Design review of the part built by this model. Coordinates are the model's own, in mm. A direction names the side the tool comes from. Round coordinates to 2 decimals unless told otherwise and drop trailing zeros. Loops run counter-clockwise (first coordinate to the right, second up) from the corner with the lowest first, then second, coordinate; pieces in that order, holes last. Notation, with made-up numbers: (59.5, 8.5) - (88.5, 8.5) arc R32 cw to (88.5, 43.5) - close; hole circle Ø9 at (-12, 44). An arc over 180 degrees is marked (long way). Answer as CSV lines item,"result". Start each with the question number.
(1) Consider section A-A (x = 11.5). Give the boundary of the cut face in (y, z).
(2) Consider section B-B (z = -3.5). Give the boundary of the cut face in (x, y).
(3) Wall thickness on L1, parallel to Z at x = -39, y = 2.75; L2, parallel to Z at x = 18, y = 3.25; L3, parallel to Z at x = 41, y = 6.75: over which ranges is each line inside the solid? List them lowest first.
(4) Consider section D-D (y = 10). Count the separate pieces of the cut face and the enclosed holes in it, and give its area (3 significant figures).
(5) For P1, Ø12, axis at x = -31, z = 2.5, coming from the +Y side; P2, Ø1.4, axis at x = -43.5, z = 0, coming from the +Y side; P3, Ø2.5, axis at x = -39.5, z = 24.5, coming from the +Y side, all flat-tipped, find the tip position at first contact; note any pin that passes through.
(6) For faces 4 (the flat face through (-6, 20, -31)), 5 (the flat face through (-44, 6, -8.5)), 6 (the flat face through (19, 8.4, 24)), 7 (the flat face through (44, 16, -7.7)), 8 (the flat face through (20, 6.4, 23)), list the 3-axis set-ups (+Z, -Z, +X, -X, +Y, -Y) from which the entire face can be reached by the end or side of a thin tool; tool diameter is ignored.
(7) Consider section C-C (x = 1.5). Give the boundary of the cut face in (y, z), and give its area (3 significant figures).
(8) Mouldability with a two-part tool opening along Z and no side actions: class faces 1 (the cylindrical face through (-36.56, 4.17, -24.86)), 2 (the flat face through (19, 8.4, -25)), 3 (the flat face through (-1, 23, -32.5)) as released by +Z, released by -Z, zero draft, split by the parting line, or undercut.
from build123d import *

# Parameters (mm, degrees)
SKETCH1_W           = 91
SKETCH1_H           = 65
BOSS_EXTRUDE1_DEPTH = 2
SKETCH2_R           = 2.5
BOSS_EXTRUDE2_DEPTH = 4.4
SKETCH3_R           = 1
BOSS_EXTRUDE3_DEPTH = 2
SKETCH4_W           = 91
SKETCH4_H           = 28
BOSS_EXTRUDE4_DEPTH = 2.8
SKETCH5_W           = 65
SKETCH5_H           = 28
SKETCH5_W_2         = 15.5
SKETCH5_H_2         = 16.5
SKETCH5_W_3         = 18
SKETCH5_H_3         = 15
BOSS_EXTRUDE5_DEPTH = 2.8
SKETCH6_W           = 91
SKETCH6_H           = 28
BOSS_EXTRUDE6_DEPTH = 2.8
SKETCH7_W           = 65
SKETCH7_H           = 28
BOSS_EXTRUDE7_DEPTH = 2.8
CHAMFER1_SIZE       = 1.5
CUT_EXTRUDE1_DEPTH  = 2.65
SKETCH11_W          = 10.5
SKETCH11_H          = 2
CUT_EXTRUDE2_DEPTH  = 3
SKETCH12_W          = 10.2
SKETCH12_H          = 1.4
CUT_EXTRUDE3_DEPTH  = 3


with BuildPart() as part:
    # Sketch1 → Boss-Extrude1 (new body)
    with BuildSketch(Plane(origin=(0, 0, 0), x_dir=(1, 0, 0), z_dir=(0, 1, 0))):
        Rectangle(SKETCH1_W, SKETCH1_H)
    extrude(amount=BOSS_EXTRUDE1_DEPTH)

    # Sketch2 → Boss-Extrude2 (add)
    with BuildSketch(Plane(origin=(0, 2, 0), x_dir=(1, 0, 0), z_dir=(0, 1, 0))):
        with Locations(Location((-39, -23.6, 0), (0, 0, 90))):
            Circle(SKETCH2_R)
        with Locations(Location((-39, 25.4, 0), (0, 0, 90))):
            Circle(SKETCH2_R)
        with Locations(Location((19, 25.4, 0), (0, 0, 90))):
            Circle(SKETCH2_R)
        with Locations(Location((19, -23.6, 0), (0, 0, 90))):
            Circle(SKETCH2_R)
    extrude(amount=BOSS_EXTRUDE2_DEPTH)

    # Sketch3 → Boss-Extrude3 (add)
    with BuildSketch(Plane(origin=(0, 6.4, 0), x_dir=(1, 0, 0), z_dir=(0, 1, 0))):
        with Locations(Location((-39, -23.6, 0), (0, 0, 270))):
            Circle(SKETCH3_R)
        with Locations(Location((-39, 25.4, 0), (0, 0, 270))):
            Circle(SKETCH3_R)
        with Locations(Location((19, 25.4, 0), (0, 0, 270))):
            Circle(SKETCH3_R)
        with Locations(Location((19, -23.6, 0), (0, 0, 270))):
            Circle(SKETCH3_R)
    extrude(amount=BOSS_EXTRUDE3_DEPTH)

    # Sketch4 → Boss-Extrude4 (add)
    with BuildSketch(Plane.XY.offset(32.5)):
        with Locations((0, 14)):
            Rectangle(SKETCH4_W, SKETCH4_H)
        with BuildLine():
            Line((-35, 14), (7.5, 14))
            ThreePointArc((7.5, 14), (15.507804885, 13.99169208), (15, 6))
            Line((15, 6), (-35, 6))
            ThreePointArc((-35, 6), (-39, 10), (-35, 14))
        make_face(mode=Mode.SUBTRACT)
    extrude(amount=-BOSS_EXTRUDE4_DEPTH)

    # Sketch5 → Boss-Extrude5 (add)
    with BuildSketch(Plane(origin=(45.5, 0, 0), x_dir=(0, 0, -1), z_dir=(1, 0, 0))):
        with Locations((0, 14)):
            Rectangle(SKETCH5_W, SKETCH5_H)
        with Locations((-18.15, 15.95)):
            Rectangle(SKETCH5_W_2, SKETCH5_H_2, mode=Mode.SUBTRACT)
        with Locations((-0.05, 15.95)):
            Rectangle(SKETCH5_W_2, SKETCH5_H_2, mode=Mode.SUBTRACT)
        with Locations((18.7, 15)):
            Rectangle(SKETCH5_W_3, SKETCH5_H_3, mode=Mode.SUBTRACT)
    extrude(amount=-BOSS_EXTRUDE5_DEPTH)

    # Sketch6 → Boss-Extrude6 (add)
    with BuildSketch(Plane(origin=(0, 0, -32.5), x_dir=(-1, 0, 0), z_dir=(0, 0, -1))):
        with Locations((0, 14)):
            Rectangle(SKETCH6_W, SKETCH6_H)
        with BuildLine():
            Line((-21.2, 20), (34.8, 20))
            ThreePointArc((34.8, 20), (36.214213562, 19.414213562), (36.8, 18))
            Line((36.8, 18), (36.8, 7))
            ThreePointArc((36.8, 7), (36.214213562, 5.585786438), (34.8, 5))
            Line((34.8, 5), (-21.2, 5))
            ThreePointArc((-21.2, 5), (-22.614213562, 5.585786438), (-23.2, 7))
            Line((-23.2, 7), (-23.2, 18))
            ThreePointArc((-23.2, 18), (-22.614213562, 19.414213562), (-21.2, 20))
        make_face(mode=Mode.SUBTRACT)
    extrude(amount=-BOSS_EXTRUDE6_DEPTH)

    # Sketch7 → Boss-Extrude7 (add)
    with BuildSketch(Plane.ZY.offset(45.5)):
        with Locations((0, 14)):
            Rectangle(SKETCH7_W, SKETCH7_H)
        with BuildLine():
            Line((-7.5, 3.5), (5.5, 3.5))
            ThreePointArc((5.5, 3.5), (6.207106781, 3.792893219), (6.5, 4.5))
            Line((6.5, 4.5), (6.5, 6.5))
            ThreePointArc((6.5, 6.5), (6.207106781, 7.207106781), (5.5, 7.5))
            Line((5.5, 7.5), (-7.5, 7.5))
            ThreePointArc((-7.5, 7.5), (-8.207106781, 7.207106781), (-8.5, 6.5))
            Line((-8.5, 6.5), (-8.5, 4.5))
            ThreePointArc((-8.5, 4.5), (-8.207106781, 3.792893219), (-7.5, 3.5))
        make_face(mode=Mode.SUBTRACT)
    extrude(amount=-BOSS_EXTRUDE7_DEPTH)

    # Chamfer1
    chamfer1_edges = [part.edges().sort_by_distance(p)[0] for p in [
        (42.7, 15, -29.7),
        (-42.7, 15, -29.7),
        (-42.7, 15, 29.7),
        (45.5, 14, 32.5),
        (-45.5, 14, 32.5),
        (-45.5, 14, -32.5),
        (45.5, 14, -32.5),
        (42.7, 15, 29.7),
    ]]
    chamfer(chamfer1_edges, length=CHAMFER1_SIZE)

    # Sketch8 → Cut-Extrude1 (cut)
    with BuildSketch(Plane(origin=(0, 28, 0), x_dir=(1, 0, 0), z_dir=(0, 1, 0))):
        Polygon((43.585786438, 31.5), (-43.585786438, 31.5), (-44.5, 30.585786438), (-44.5, -30.585786438), (-43.585786438, -31.5), (43.585786438, -31.5), (44.5, -30.585786438), (44.5, 30.585786438), align=None)
    extrude(amount=-CUT_EXTRUDE1_DEPTH, mode=Mode.SUBTRACT)

    # Sketch11 → Cut-Extrude2 (cut)
    with BuildSketch(Plane(origin=(-42.7, 0, 0), x_dir=(0, 0, -1), z_dir=(1, 0, 0))):
        with Locations((0.15, 21.1)):
            Rectangle(SKETCH11_W, SKETCH11_H)
    extrude(amount=-CUT_EXTRUDE2_DEPTH, mode=Mode.SUBTRACT)

    # Sketch12 → Cut-Extrude3 (cut)
    with BuildSketch(Plane(origin=(45.5, 0, 0), x_dir=(0, 0, -1), z_dir=(1, 0, 0))):
        with Locations((-21.2, 26.05)):
            Rectangle(SKETCH12_W, SKETCH12_H)
        with Locations((21.4, 26.05)):
            Rectangle(SKETCH12_W, SKETCH12_H)
    extrude(amount=-CUT_EXTRUDE3_DEPTH, mode=Mode.SUBTRACT)


solid = part.part
Determined:
1,outline,"(0, -32.5) - (5, -32.5) - (5, -29.7) - (2, -29.7) - (2, 29.7) - (6, 29.7) - (6, 32.5) - (0, 32.5) - close; (15.73, 29.7) - (25.35, 29.7) - (25.35, 31.5) - (28, 31.5) - (28, 32.5) - (15.73, 32.5) - close; (20, -32.5) - (28, -32.5) - (28, -31.5) - (25.35, -31.5) - (25.35, -29.7) - (20, -29.7) - close"
2,outline,"(-45.5, 0) - (45.5, 0) - (45.5, 7.7) - (42.7, 7.7) - (42.7, 2) - (-42.7, 2) - (-42.7, 3.5) - (-45.5, 3.5) - close; (-45.5, 7.5) - (-42.7, 7.5) - (-42.7, 20.1) - (-45.5, 20.1) - close; (-45.5, 22.1) - (-42.7, 22.1) - (-42.7, 25.35) - (-44.5, 25.35) - (-44.5, 28) - (-45.5, 28) - close; (42.7, 24.2) - (45.5, 24.2) - (45.5, 28) - (44.5, 28) - (44.5, 25.35) - (42.7, 25.35) - close"
3,L1,"z = -32.5 to -29.7, -27.9 to -22.9, 21.1 to 26.1, 29.7 to 32.5"
3,L2,"z = -32.5 to -29.7, -27.69 to -23.11, 21.31 to 25.89, 29.7 to 32.5"
3,L3,"z = -32.5 to -29.7, 29.7 to 32.5"
4,separate pieces,"5"
4,enclosed holes,"0"
4,area,"380 mm^2"
5,P1,"stops at y = 2"
5,P2,"stops at y = 25.35"
5,P3,"stops at y = 8.4"
6,face 4,"-Z"
6,face 5,"-X"
6,face 6,"-Z, +X, +Y"
6,face 7,"+X"
6,face 8,"+Y"
7,outline,"(0, -32.5) - (5, -32.5) - (5, -29.7) - (2, -29.7) - (2, 29.7) - (6, 29.7) - (6, 32.5) - (0, 32.5) - close; (14, 29.7) - (25.35, 29.7) - (25.35, 31.5) - (28, 31.5) - (28, 32.5) - (14, 32.5) - close; (20, -32.5) - (28, -32.5) - (28, -31.5) - (25.35, -31.5) - (25.35, -29.7) - (20, -29.7) - close"
7,area,"202 mm^2"
8,face 1,"undercut"
8,face 2,"zero draft"
8,face 3,"released by -Z"
